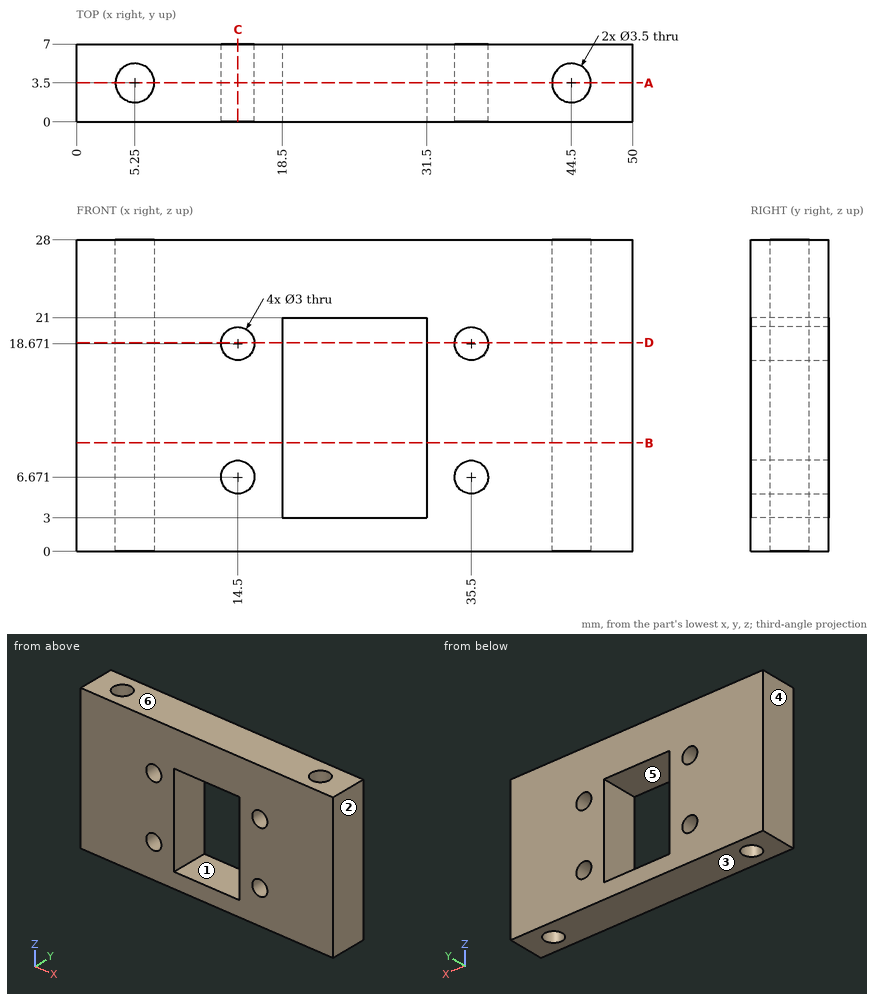
Answer from the drawing. Dimensions are ordinates in mm from the lowest x, y and z of the part. A direction names the side the tool comes from. Round coordinates to 2 decimals unless told otherwise and drop trailing zeros. Write each loop counter-clockwise with the first axis right and the second up, starting at its lowest first coordinate (ties: lowest second). Pieces come first, ordered by that corner, then holes.
1. Given pin 1 Ø3 at (x, y) = (44.5, 3.5) entering from +Z, flat-ended and moving along its own axis, determine where the tip first touches the part or whether it passes through.
2. The part is cut by section B-B, the plane z = 9.75. Determine the outline of the cut face in (x, y), then the cut area to 3 significant figures.
3. Determine the mould class of the marked faces 3, 4, 5 and 6 for opening direction Z: pulls with the +Z half, pulls with the -Z half, needs draft (parallel to the pull), parting line crosses it, or undercut.
4. The part is cut by section A-A, the plane y = 3.5. Determine the outline of the cut face in (x, z).
5. The part is cut by section D-D, the plane z = 18.75. Determine the outline of the cut face in (x, y), then the cut area to 3 significant figures.
6. Which of the six approach directions +Z, -Z, +X, -X, +Y, -Y give full straight-line access (tool end or side, diameter ignored) to the marked faces 1 and 2?
7. The part is cut by section C-C, the plane x = 14.5. Determine the outline of the cut face in (y, z).
8. Straight lines are drawn through the part: L1, parallel to X at y = 1.5, z = 8.5; L2, parallel to X at y = 4, z = 3.75; L3, parallel to Z at x = 29, y = 5. For each, find the intervals that lie inside material, in ascending order.
Values:
1. pin 1: passes through
2. outline: (0, 0) - (18.5, 0) - (18.5, 7) - (0, 7) - close; (31.5, 0) - (50, 0) - (50, 7) - (31.5, 7) - close; hole circle Ø3.5 at (5.25, 3.5); hole circle Ø3.5 at (44.5, 3.5)
2. area: 240 mm2
3. face 3: pulls with the -Z half
3. face 4: needs draft
3. face 5: undercut
3. face 6: pulls with the +Z half
4. outline: (0, 0) - (3.5, 0) - (3.5, 28) - (0, 28) - close; (7, 0) - (42.75, 0) - (42.75, 28) - (7, 28) - close; (46.25, 0) - (50, 0) - (50, 28) - (46.25, 28) - close; hole circle Ø3 at (14.5, 6.67); hole circle Ø3 at (14.5, 18.67); hole (18.5, 3) - (31.5, 3) - (31.5, 21) - (18.5, 21) - close; hole circle Ø3 at (35.5, 6.67); hole circle Ø3 at (35.5, 18.67)
5. outline: (0, 0) - (13, 0) - (13, 7) - (0, 7) - close; (16, 0) - (18.5, 0) - (18.5, 7) - (16, 7) - close; (31.5, 0) - (34, 0) - (34, 7) - (31.5, 7) - close; (37, 0) - (50, 0) - (50, 7) - (37, 7) - close; hole circle Ø3.5 at (5.25, 3.5); hole circle Ø3.5 at (44.5, 3.5)
5. area: 198 mm2
6. face 1: +Y, -Y
6. face 2: +Z, -Z, +X, +Y, -Y
7. outline: (0, 0) - (7, 0) - (7, 5.17) - (0, 5.17) - close; (0, 8.17) - (7, 8.17) - (7, 17.17) - (0, 17.17) - close; (0, 20.17) - (7, 20.17) - (7, 28) - (0, 28) - close
8. L1: x = 0 to 18.5, 31.5 to 50
8. L2: x = 0 to 3.57, 6.93 to 18.5, 31.5 to 42.82, 46.18 to 50
8. L3: z = 0 to 3, 21 to 28
